Read the model definition and answer for the solid it produces. Units are mm, in the model's axes. A direction names the side the tool comes from. Give positions to 0.01 mm unless a question says otherwise; leave off trailing zeros. Write each loop counter-clockwise with the first axis right and the second up, starting at its lowest first coordinate (ties: lowest second). Pieces come first, ordered by that corner, then holes. Notation, with made-up numbers: M 85,-13 L 134,-13 A27 ccw 134,19 Z; hole C 82,70 d8. An arc over 180 degrees is marked long. Use a Markdown table: item, result. Add a question column.
Item 1: Consider probe 1 along Y at (x, z) = (7, 94) (3 decimals); probe 2 along Y at (x, z) = (4.5, 7.5). Determine where each line is inside the solid, lowest interval first. Write a range as [from, to].
Item 2: A cutting plane is placed at A-A on z = 107.5. Determine the outline of the cut face in (x, y) (3 decimals), then the cut area to 3 significant figures.
Item 3: A cutting plane is placed at B-B on x = 6.25. Determine the outline of the cut face in (y, z) (3 decimals), then the cut area to 3 significant figures.
Item 4: Given P1, Ø3, axis at y = 8.5, z = 44, coming from the +X side (3 decimals), flat-ended and moving along its own axis, determine where the tip first touches the part or whether it passes through.
Item 5: For faces 1 (the flat face through (3.175, 10, 59)), 2 (the flat face through (1.675, 10, 59)), determine the directions among +Z, -Z, +X, -X, +Y, -Y from which every point of the face is accessible in a straight line to the end or side of a thin tool.
from build123d import *

# Parameters (mm, degrees)
BOSS_EXTRUDE1_DEPTH    = 120
CONVERT_SOLID1_DEPTH   = 120
CONVERT_SOLID1_2_DEPTH = 120


# Read off the part's stored shape, not the designer's step: Convert-Solid1
with BuildPart() as part:
    # Sketch1 → Boss-Extrude1 (new body)
    with BuildSketch(Plane.XY):
        Polygon((0, 15), (0, 0), (10, 0), (10, 3.175), (3.175, 3.175), (3.175, 15), align=None)
    extrude(amount=BOSS_EXTRUDE1_DEPTH)

    # Convert-Solid1 outline → Convert-Solid1 (cut)
    with BuildSketch(Plane.XY):
        with BuildLine():
            Line((1.675, 5.175), (1.675, 15))
            Line((1.675, 15), (0, 15))
            Line((0, 15), (0, 0))
            Line((0, 0), (10, 0))
            Line((10, 0), (10, 1.675))
            Line((10, 1.675), (5.175, 1.675))
            ThreePointArc((5.175, 1.675), (2.700126266, 2.700126266), (1.675, 5.175))
        make_face()
    extrude(amount=CONVERT_SOLID1_DEPTH, mode=Mode.SUBTRACT)

    # Convert-Solid1 2 outline → Convert-Solid1 2 (add)
    with BuildSketch(Plane.XY):
        with BuildLine():
            ThreePointArc((5.175, 3.175), (3.760786438, 3.760786438), (3.175, 5.175))
            Line((3.175, 5.175), (3.175, 3.175))
            Line((3.175, 3.175), (5.175, 3.175))
        make_face()
    extrude(amount=CONVERT_SOLID1_2_DEPTH)


solid = part.part
Filled in:
| question | item | result |
|---|---|---|
| 1 | probe 1 | [1.675, 3.175] |
| 1 | probe 2 | [1.74, 3.29] |
| 2 | outline | M 1.675,5.175 A3.5 ccw 5.175,1.675 L 10,1.675 L 10,3.175 L 5.175,3.175 A2 cw 3.175,5.175 L 3.175,15 L 1.675,15 Z |
| 2 | area | 28.5 mm² |
| 3 | outline | M 1.675,0 L 3.175,0 L 3.175,120 L 1.675,120 Z |
| 3 | area | 180 mm² |
| 4 | P1 | x = 3.175 |
| 5 | face 1 | +Z, -Z, +X, +Y |
| 5 | face 2 | +Z, -Z, -X, +Y, -Y |
